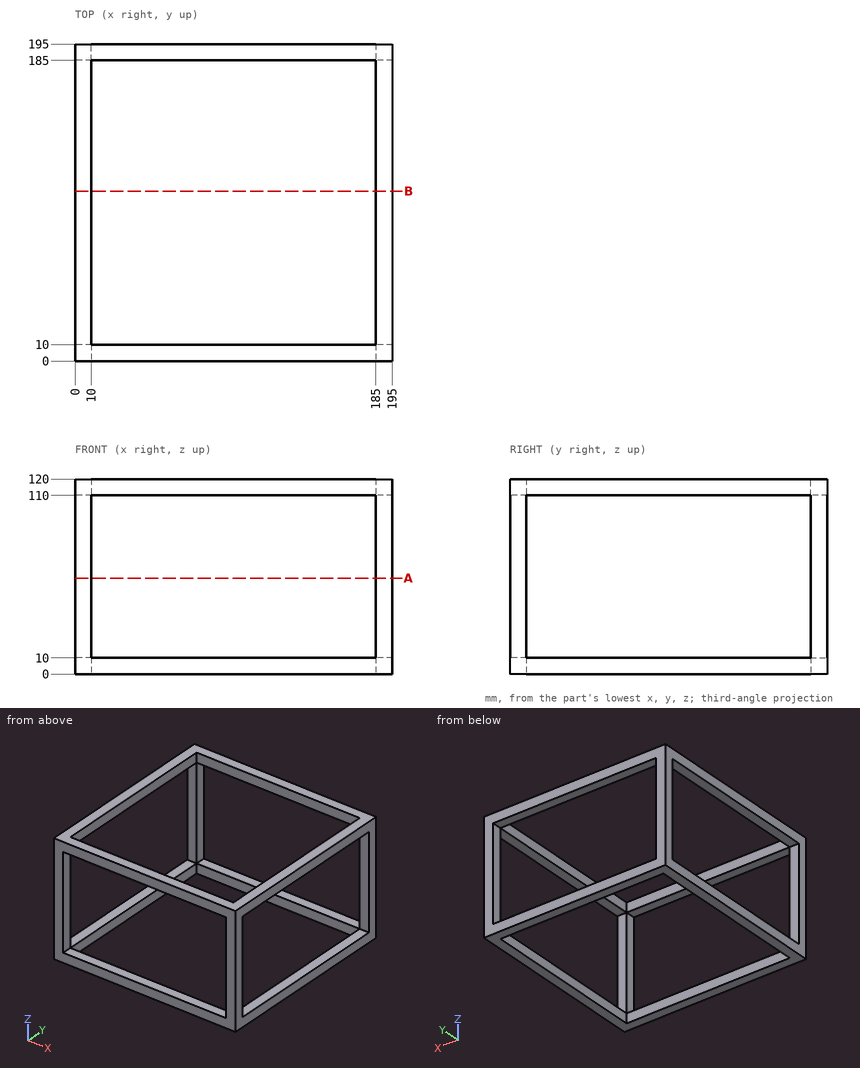
Print and shaded views of the part. All mm, measured from the part's lowest x, y and z. Round coordinates to 2 decimals unless told otherwise and drop trailing zeros. Order: outer loops, then holes, each group sorted by start corner. A loop starts at its lowest first (then second) coordinate and runs counter-clockwise, first axis right, second up.
Q1. Wall check: L1, parallel to X at y = 66, z = 113.5. Give the ranges that are in metal, low to high.
Q2. Drop a flat-ended pin along its axis: pin 1 (8 mm diameter, centred on x = 6.5, z = 69, fed in from -Y). Give the stop position or say it passes through.
Q3. Slice it at A-A (z = 59). Write the cut outline in (x, y), and give its area (3 significant figures).
Q4. Slice it at B-B (y = 104.5). Write the cut outline in (x, z), and give its area (3 significant figures).
Results below:
1. L1: x = 0 to 10, 185 to 195
2. pin 1: stops at y = 0
3. outline: (0, 0) - (10, 0) - (10, 10) - (0, 10) - close; (0, 185) - (10, 185) - (10, 195) - (0, 195) - close; (185, 0) - (195, 0) - (195, 10) - (185, 10) - close; (185, 185) - (195, 185) - (195, 195) - (185, 195) - close
3. area: 400 mm2
4. outline: (0, 0) - (10, 0) - (10, 10) - (0, 10) - close; (0, 110) - (10, 110) - (10, 120) - (0, 120) - close; (185, 0) - (195, 0) - (195, 10) - (185, 10) - close; (185, 110) - (195, 110) - (195, 120) - (185, 120) - close
4. area: 400 mm2
